The listing builds one solid part. Answer for the finished solid, in the listing's coordinates (mm). A direction names the side the tool comes from. Round coordinates to 2 decimals unless told otherwise and drop trailing zeros. Loops run counter-clockwise (first coordinate to the right, second up) from the corner with the lowest first, then second, coordinate; pieces in that order, holes last. Notation, with made-up numbers: M -30,-27.75 L -13,-27.75 A26 ccw -13,4.25 Z; hole C -24.75,-10.5 d7. An arc over 180 degrees is marked long. Answer as a JSON object with one key per item and string values.
Autodesk Inventor part; units mm, degrees
ref_plane "YZ Plane" through (0, 0, 0) normal (1, 0, 0) x (0, 1, 0)
ref_plane "XZ Plane" through (0, 0, 0) normal (0, 1, 0) x (-1, 0, 0)
ref_plane "XY Plane" through (0, 0, 0) normal (0, 0, 1) x (1, 0, 0)
sketch "Sketch1" plane through (0, 0, 0) normal (0, 0, 1) x (1, 0, 0)
  line L0 (-35.56, 0) -> (35.56, 0)
  line L1 (0, -20.0025) -> (0, 20.0025)
  line L2 (-25.4, 12.7) -> (25.4, 12.7)
  line L3 (25.4, 12.7) -> (25.4, -12.7)
  line L4 (25.4, -12.7) -> (-25.4, -12.7)
  line L5 (-25.4, -12.7) -> (-25.4, 12.7)
  circle A0 centre (0, 0) radius 14.2875 construction
  point P0 (-25.4, 0)
  point P1 (0, 12.7)
  dimension "d0" = 28.575
  dimension "d1" = 50.8
  dimension "d2" = 25.4
extrude "Extrusion1" add sketch "Sketch1" along normal blind 9.525
sketch "Sketch2" plane through (-25.4, 12.7, 0) normal (0, 1, 0) x (1, 0, 0)
  line L0 (0, -9.525) -> (50.8, -9.525)
  line L1 (0, 0) -> (50.8, 0)
  line L2 (0, 0) -> (0, -9.525)
  line L3 (44.45, 0) -> (44.45, -1.905)
  line L4 (6.35, -1.905) -> (6.35, 0)
  line L5 (6.35, -1.905) -> (44.45, -1.905)
  line L6 (25.4, 0) -> (25.4, -9.525) construction
  dimension "d5" = 6.35
  dimension "d7" = 1.905
extrude "Extrusion2" cut sketch "Sketch2" against normal through all
sketch "Sketch3" plane through (0, 0, 0) normal (0, 0, -1) x (-1, 0, 0)
  line L0 (25.4, 12.7) -> (19.05, 12.7)
  line L1 (35.56, 0) -> (-35.56, 0)
  line L2 (0, -17.78) -> (0, 17.78)
  point P0 (0, 0)
  point P1 (22.225, 7.9375)
  point P2 (22.225, -7.9375)
  point P3 (22.225, 12.7)
  dimension "d10" = 4.7625
hole "Hole1" at (-22.225, 7.9375, 0) at (-22.225, -7.9375, 0) direction (0, 0, 1) diameter 3.683 depth 6.35 tip angle 118
mirror "Mirror1" about plane through (0, 0, 0) normal (1, 0, 0) of "Hole1"
sketch "Sketch4" plane through (0, 0, 9.525) normal (0, 0, 1) x (1, 0, 0)
  point P0 (0, 0)
  point P1 (0, 0)
hole "Hole2" at (0, 0, 9.525) direction (0, 0, -1) diameter 8.6614 end through all
properties part number "encoder mount"
Item 1: Straight lines are drawn through the part: line 1 (Y direction, x = 0, z = 6.5); line 2 (X direction, y = -3.25, z = 1.25); line 3 (X direction, y = 0, z = 4). For each, find the intervals that lie inside material, in ascending order.
Values follow:
{"line 1": "-12.7 to -4.33, 4.33 to 12.7", "line 2": "-25.4 to -19.05, 19.05 to 25.4", "line 3": "-25.4 to -4.33, 4.33 to 25.4"}
Item 2: The part is cut by section A-A (x = 0). Give the vertices of the cut face in (y, z) (3 decimals), then the cut area to 3 significant figures.
Values follow:
{"outline": "M -12.7,1.905 L -4.331,1.905 L -4.331,9.525 L -12.7,9.525 Z; M 4.331,1.905 L 12.7,1.905 L 12.7,9.525 L 4.331,9.525 Z", "area": "128 mm^2"}
Item 3: Determine the mould class of faces 4 (the face through (5, 0, 9.525)), 5 (the face through (-5, 0, 1.905)), 6 (the face through (25.4, 0, 5)) for opening direction X: released by +X, released by -X, zero draft, split by the parting line, or undercut.
Values follow:
{"face 4": "zero draft", "face 5": "undercut", "face 6": "released by +X"}
Item 4: Which of the six approach directions +Z, -Z, +X, -X, +Y, -Y give full straight-line access (tool end or side, diameter ignored) to faces 1 (the face through (-19.05, 0, 1)), 2 (the face through (24.023, 7.538, 3.219)), 3 (the face through (0, 12.7, 6))?
Values follow:
{"face 1": "-Z, +Y, -Y", "face 2": "-Z", "face 3": "+Z, -Z, +X, -X, +Y"}
Item 5: The part is cut by section B-B (y = 0). Give the vertices of the cut face in (x, z) (3 decimals).
Values follow:
{"outline": "M -25.4,0 L -19.05,0 L -19.05,1.905 L -4.331,1.905 L -4.331,9.525 L -25.4,9.525 Z; M 4.331,1.905 L 19.05,1.905 L 19.05,0 L 25.4,0 L 25.4,9.525 L 4.331,9.525 Z"}
Item 6: The part is cut by section C-C (z = 3.5). Give the vertices of the cut face in (x, y) (1 decimal), then the cut area to 3 significant figures.
Values follow:
{"outline": "M -25.4,-12.7 L 25.4,-12.7 L 25.4,12.7 L -25.4,12.7 Z; hole C -22.2,-7.9 d3.7; hole C -22.2,7.9 d3.7; hole C 0,0 d8.7; hole C 22.2,-7.9 d3.7; hole C 22.2,7.9 d3.7", "area": "1,190 mm^2"}
Item 7: A flat-ended cylindrical pin translates along its axis: P1, Ø8, axis at x = -4, y = -6, coming from the -Z side (3 decimals). Find the tip coordinate at first contact, or state that the pin passes through.
Values follow:
{"P1": "z = 1.905"}
Item 8: The part is cut by section D-D (z = 1). Give the number of separate pieces and of enclosed holes in the cut face, then the cut area to 3 significant figures.
Values follow:
{"separate pieces": "2", "enclosed holes": "4", "area": "280 mm^2"}
